from build123d import *

# Parameters (mm, degrees)
F0_R     = 0.75
F1_DEPTH = 3


with BuildPart() as f1:
    # F0 (on Front) → F1 (new body)
    with BuildSketch(Plane.XZ):
        with BuildLine():
            ThreePointArc((2, 3), (0, 5), (-2, 3))
            Line((-2, 3), (-2, -3))
            ThreePointArc((-2, -3), (0, -5), (2, -3))
            Line((2, -3), (2, 3))
        make_face()
        with Locations((0, -3)):
            Circle(F0_R, mode=Mode.SUBTRACT)
        Circle(F0_R, mode=Mode.SUBTRACT)
        with Locations((0, 3)):
            Circle(F0_R, mode=Mode.SUBTRACT)
    extrude(amount=F1_DEPTH)


solid = f1.part
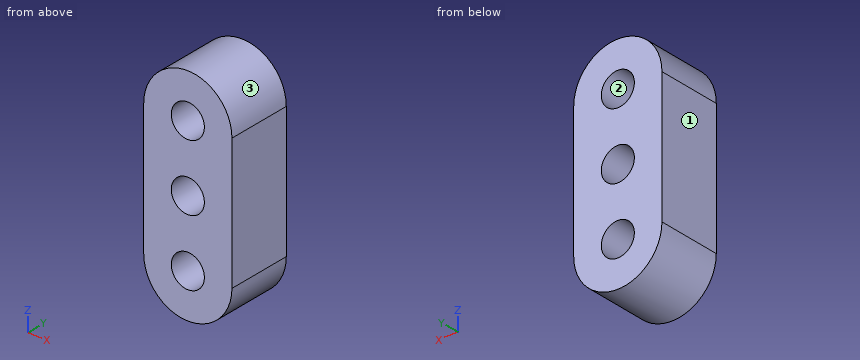
Work out the finished part from the listing and answer in its coordinate system (mm). Face numbers are marked on the shaded views. Give positions to 0.01 mm unless a question says otherwise; leave off trailing zeros. Write each loop counter-clockwise with the first axis right and the second up, starting at its lowest first coordinate (ties: lowest second). Pieces come first, ordered by that corner, then holes.
Q1. Straight lines are drawn through the part: L1, parallel to Z at x = 0, y = -1.25; L2, parallel to Z at x = -0.55, y = -2.8; L3, parallel to X at y = -0.15, z = 0.5. For each, find the intervals that lie inside material, in ascending order.
Answer:
L1: z = -5 to -3.75, -2.25 to -0.75, 0.75 to 2.25, 3.75 to 5
L2: z = -4.92 to -3.51, -2.49 to -0.51, 0.51 to 2.49, 3.51 to 4.92
L3: x = -2 to -0.56, 0.56 to 2
Q2. Given pin 1 (2 mm diameter, centred on x = 0.5, z = 0, fed in from -Y); pin 2 (1.4 mm diameter, centred on x = 0, z = 3, fed in from -Y), each flat-ended and moving along its own axis, determine where each tip first touches the part or whether it passes through.
Answer:
pin 1: stops at y = -3
pin 2: passes through
Q3. For a pull along X with two mould halves and no side action, classify the marked faces 1, 2 and 3 as released by +X, released by -X, zero draft, split by the parting line, or undercut.
Answer:
face 1: released by -X
face 2: undercut
face 3: split by the parting line
Q4. The part is cut by section C-C on z = 2.75. Give the vertices of the cut face in (x, y).
Answer:
outline: (-2, -3) - (-0.71, -3) - (-0.71, 0) - (-2, 0) - close; (0.71, -3) - (2, -3) - (2, 0) - (0.71, 0) - close
Q5. The part is cut by section D-D on x = 0.65. Give the vertices of the cut face in (y, z).
Answer:
outline: (-3, -4.89) - (0, -4.89) - (0, -3.37) - (-3, -3.37) - close; (-3, -2.63) - (0, -2.63) - (0, -0.37) - (-3, -0.37) - close; (-3, 0.37) - (0, 0.37) - (0, 2.63) - (-3, 2.63) - close; (-3, 3.37) - (0, 3.37) - (0, 4.89) - (-3, 4.89) - close
Q6. The part is cut by section B-B on y = -2.65. Give the vertices of the cut face in (x, z), and give its area (3 significant figures).
Answer:
outline: (-2, -3) arc R2 ccw to (2, -3) - (2, 3) arc R2 ccw to (-2, 3) - close; hole circle Ø1.5 at (0, -3); hole circle Ø1.5 at (0, 0); hole circle Ø1.5 at (0, 3)
area: 31.3 mm2
Q7. The part is cut by section A-A on x = 0. Give the vertices of the cut face in (y, z).
Answer:
outline: (-3, -5) - (0, -5) - (0, -3.75) - (-3, -3.75) - close; (-3, -2.25) - (0, -2.25) - (0, -0.75) - (-3, -0.75) - close; (-3, 0.75) - (0, 0.75) - (0, 2.25) - (-3, 2.25) - close; (-3, 3.75) - (0, 3.75) - (0, 5) - (-3, 5) - close
